Could you check a few things on this model? Use its own coordinates, in mm. A direction names the side the tool comes from. Give positions to 0.01 mm unless a question says otherwise; leave off trailing zeros. Loops run counter-clockwise (first coordinate to the right, second up) from the corner with the lowest first, then second, coordinate; pieces in that order, holes last. Notation, with made-up numbers: (43.5, -30.75) - (94.5, -30.75) arc R13 ccw to (94.5, -21.75) - close; hole circle Ø2 at (72, -2.5). An arc over 180 degrees is marked (long way). Write each question's results on one line, items separated by ' | '. Start each with the question number.
(1) If we mould it in two halves opening along X, with no side actions, what happens to faces 3 (the face through (0, -43.942, 27)), 4 (the face through (33.463, -24.783, -24.332)), 5 (the face through (35.24, -24.783, 26.147))? For each: released by +X, released by -X, zero draft, split by the parting line, or undercut.
(2) On a 3-axis mill with a long thin cutter (end or side, diameter ignored), from which of +Z, -Z, +X, -X, +Y, -Y can I reach the whole of each face in a straight line? I mean faces 1 (the face through (35.32, -1.53, 0.32)), 2 (the face through (-15, -2.54, 15)). Say none if no direction works.
(3) I need wall thicknesses on line 1 (Z direction, x = 0, y = -21.5); line 2 (Z direction, x = 31, y = -38); line 3 (Z direction, x = 7, y = -24). Which ranges of each line are inside material? Lowest first, please.
(4) For pin 1 (10 mm diameter, centred on x = 16.5, z = -14.5, fed in from -Y), with a flat end and sliding along its axis, tell me the tip position at first contact or that it passes through.
(5) Suppose I cut it at A-A (y = -33.5). Please give me the cut outline in (x, z).
(6) Suppose I cut it at C-C (z = 0). Please give me the cut outline in (x, y), and give its area (3 significant figures).
(7) Suppose I cut it at D-D (x = 26.5). Please give me the cut outline in (y, z), and give its area (3 significant figures).
(8) Suppose I cut it at B-B (x = 0). Please give me the cut outline in (y, z).
from build123d import *

# Parameters (mm, degrees)
F0_W     = 73.534466
F0_H     = 55.191916
F0_R     = 15.396007
F1_DEPTH = 43.942
F2_R     = 5.08
F3_T     = -2.54


with BuildPart() as f1:
    # F0 (on Front) → F1 (new body)
    with BuildSketch(Plane.XZ):
        Rectangle(F0_W, F0_H)
        Circle(F0_R, mode=Mode.SUBTRACT)
    extrude(amount=F1_DEPTH)

    # F2
    f2_edges = [f1.edges().sort_by_distance(p)[0] for p in [
        (36.767233, 0, 0),
        (0, 0, 27.595958),
        (-36.767233, 0, 0),
        (0, 0, -27.595958),
        (-15.396007, 0, 0),
        (-36.767233, -21.971, -27.595958),
        (36.767233, -21.971, -27.595958),
        (36.767233, -21.971, 27.595958),
        (-36.767233, -21.971, 27.595958),
    ]]
    fillet(f2_edges, radius=F2_R)

    # F3
    f3_openings = [f1.faces().sort_by_distance(p)[0] for p in [
        (35.847806, -43.942, 0),
    ]]
    offset(amount=F3_T, openings=f3_openings)


solid = f1.part
Output values:
1) face 3: zero draft | face 4: undercut | face 5: released by +X
2) face 1: +Z, -Z, +X, +Y | face 2: -Y
3) line 1: -27.6 to -25.06, -17.94 to -15.4, 15.4 to 17.94, 25.06 to 27.6 | line 2: -27.6 to -25.06, 25.06 to 27.6 | line 3: -27.6 to -25.06, -16.51 to -13.71, 13.71 to 16.51, 25.06 to 27.6
4) pin 1: y = -43.94
5) outline: (-36.77, -22.52) arc R5.08 ccw to (-31.69, -27.6) - (31.69, -27.6) arc R5.08 ccw to (36.77, -22.52) - (36.77, 22.52) arc R5.08 ccw to (31.69, 27.6) - (-31.69, 27.6) arc R5.08 ccw to (-36.77, 22.52) - close; circle Ø35.87 at (0, 0); hole (-34.23, -22.52) arc R2.54 ccw to (-31.69, -25.06) - (31.69, -25.06) arc R2.54 ccw to (34.23, -22.52) - (34.23, 22.52) arc R2.54 ccw to (31.69, 25.06) - (-31.69, 25.06) arc R2.54 ccw to (-34.23, 22.52) - close; hole circle Ø30.79 at (0, 0)
6) outline: (-36.77, -43.94) - (-34.23, -43.94) - (-34.23, -5.08) arc R2.54 cw to (-31.69, -2.54) - (-20.48, -2.54) arc R2.54 cw to (-17.94, -5.08) - (-17.94, -43.94) - (-15.4, -43.94) - (-15.4, -5.08) arc R5.08 ccw to (-20.48, 0) - (-31.69, 0) arc R5.08 ccw to (-36.77, -5.08) - close; (15.4, -43.94) - (17.94, -43.94) - (17.94, -5.08) arc R2.54 cw to (20.48, -2.54) - (31.69, -2.54) arc R2.54 cw to (34.23, -5.08) - (34.23, -43.94) - (36.77, -43.94) - (36.77, -5.08) arc R5.08 ccw to (31.69, 0) - (20.48, 0) arc R5.08 ccw to (15.4, -5.08) - close | area: 513 mm2
7) outline: (-43.94, -27.6) - (-5.08, -27.6) arc R5.08 ccw to (0, -22.52) - (0, 22.52) arc R5.08 ccw to (-5.08, 27.6) - (-43.94, 27.6) - (-43.94, 25.06) - (-5.08, 25.06) arc R2.54 cw to (-2.54, 22.52) - (-2.54, -22.52) arc R2.54 cw to (-5.08, -25.06) - (-43.94, -25.06) - close | area: 342 mm2
8) outline: (-43.94, -27.6) - (-5.08, -27.6) arc R5.08 ccw to (0, -22.52) - (0, -20.48) arc R5.08 ccw to (-5.08, -15.4) - (-43.94, -15.4) - (-43.94, -17.94) - (-5.08, -17.94) arc R2.54 cw to (-2.54, -20.48) - (-2.54, -22.52) arc R2.54 cw to (-5.08, -25.06) - (-43.94, -25.06) - close; (-43.94, 15.4) - (-5.08, 15.4) arc R5.08 ccw to (0, 20.48) - (0, 22.52) arc R5.08 ccw to (-5.08, 27.6) - (-43.94, 27.6) - (-43.94, 25.06) - (-5.08, 25.06) arc R2.54 cw to (-2.54, 22.52) - (-2.54, 20.48) arc R2.54 cw to (-5.08, 17.94) - (-43.94, 17.94) - close
